Autodesk Inventor part; units mm, degrees
ref_plane "YZ Plane" through (0, 0, 0) normal (1, 0, 0) x (0, 1, 0)
ref_plane "XZ Plane" through (0, 0, 0) normal (0, 1, 0) x (-1, 0, 0)
ref_plane "XY Plane" through (0, 0, 0) normal (0, 0, 1) x (1, 0, 0)
sketch "Sketch1" plane through (0, 0, 0) normal (0, 0, 1) x (1, 0, 0)
  line L0 (-1.6583, -2.5) -> (1.6583, -2.5)
  arc A0 (1.6583, -2.5) -> (-1.6583, -2.5) centre (0, 0) ccw
  arc A1 (2.2111, -3.3333) -> (-2.2111, -3.3333) centre (0, 0) ccw
  line L1 (2.2111, -3.3333) -> (-2.2111, -3.3333)
  dimension "d0" = 1
  dimension "d1" = 3
  dimension "d2" = 3.3166
  dimension "d3" = 0.8333
  dimension "d4" = 3.3333
  dimension "d5" = 3.3333
  dimension "d6" = 4
  dimension "d7" = 0
extrude "Extrusion1" add sketch "Sketch1" along normal blind 12
sketch "Sketch2" plane through (0, 0, 12) normal (0, 0, 1) x (1, 0, 0)
  arc A0 (2.2111, -3.3333) -> (-2.2111, -3.3333) centre (0, 0) ccw
  line L0 (-2.2111, -3.3333) -> (2.2111, -3.3333)
extrude "Extrusion2" add sketch "Sketch2" against normal blind 6.35
sketch "Sketch3" plane through (0, 0, 12) normal (0, 0, 1) x (1, 0, 0)
  point P0 (0, 0)
hole "Hole1" at (0, 0, 12) direction (0, 0, -1) diameter 2.6416 end through all
properties part number "ShaftD6Female-632Female"
Verification items for the finished model (mm, model axes). A direction names the side the tool comes from. Give positions to 0.01 mm unless a question says otherwise; leave off trailing zeros. Loops run counter-clockwise (first coordinate to the right, second up) from the corner with the lowest first, then second, coordinate; pieces in that order, holes last.
1. Thickness scan on line 1 (Y direction, x = 0, z = 8.25); line 2 (Y direction, x = 0, z = 1.35); line 3 (X direction, y = 0, z = 9.5). Record the ranges inside material, lowest first.
2. Set-up check for faces 1 (the flat face through (0, 2, 5.65)), 2 (the flat face through (-0.9, 1.2, 12)): record each of +Z, -Z, +X, -X, +Y, -Y from which the full face is reachable in a straight line by a thin tool's end or side.
3. Section check D-D, the plane x = 2.5. Enter the section's corners in (y, z).
4. Section check C-C, the plane z = 4.5. Enter the section's corners in (x, y), then the cut area to 3 significant figures.
5. Section check B-B, the plane y = 0. Enter the section's corners in (x, z), then the cut area to 3 significant figures.
6. Go/stop test with flat-tipped pins: pin 1 Ø4 at (y, z) = (-1, 9) entering from +X; pin 2 Ø1.6 at (x, y) = (1, -1) entering from -Z; pin 3 Ø1.5 at (x, z) = (-3, 6) entering from -Y; pin 4 Ø1 at (x, z) = (1, 2) entering from +Y. Record where each tip stops, or that it passes through.
7. Section check A-A, the plane x = 0. Enter the section's corners in (y, z).
8. Mould release check, pull along Y, two halves, no side actions. Record for faces 3 (the flat face through (0, -3, 0)), 4 (the cylindrical face through (0.8, 1.05, 8.78)), 5 (the cylindrical face through (0, 4, 6)), 6 (the flat face through (0, -3.333, 6)): released by +Y, released by -Y, zero draft, split by the parting line, or undercut.
Geometry says:
1. line 1: y = -3.33 to -1.32, 1.32 to 4
1. line 2: y = -3.33 to -2.5, 3 to 4
1. line 3: x = -4 to -1.32, 1.32 to 4
2. face 1: -Z
2. face 2: +Z, +X, -X, +Y, -Y
3. outline: (-3.12, 0) - (-1.66, 0) - (-1.66, 5.65) - (1.66, 5.65) - (1.66, 0) - (3.12, 0) - (3.12, 12) - (-3.12, 12) - close
4. outline: (-2.21, -3.33) - (2.21, -3.33) arc R4 ccw (long way) to start; hole (-1.66, -2.5) - (1.66, -2.5) arc R3 ccw (long way) to start
4. area: 21.1 mm2
5. outline: (-4, 0) - (-3, 0) - (-3, 5.65) - (-1.32, 5.65) - (-1.32, 12) - (-4, 12) - close; (1.32, 5.65) - (3, 5.65) - (3, 0) - (4, 0) - (4, 12) - (1.32, 12) - close
5. area: 45.3 mm2
6. pin 1: stops at x = 4
6. pin 2: stops at z = 5.65
6. pin 3: stops at y = -3.31
6. pin 4: stops at y = 3.97
7. outline: (-3.33, 0) - (-2.5, 0) - (-2.5, 5.65) - (-1.32, 5.65) - (-1.32, 12) - (-3.33, 12) - close; (1.32, 5.65) - (3, 5.65) - (3, 0) - (4, 0) - (4, 12) - (1.32, 12) - close
8. face 3: zero draft
8. face 4: undercut
8. face 5: split by the parting line
8. face 6: released by -Y
